CAD build for the part. Positions are in the model's coordinates, mm. Coordinates: 2 decimals unless noted, no trailing zeros. Loops run counter-clockwise (first coordinate to the right, second up) from the corner with the lowest first, then second, coordinate; pieces in that order, holes last. Notation, with made-up numbers: (16.25, -33.75) -> (49.25, -33.75) arc R16 ccw to (49.25, -26.75) -> close; hole circle Ø4 at (51.25, 31). An arc over 180 degrees is marked (long way). Answer as a JSON object with one key per item and string values. Group by question number.
from build123d import *

# Parameters (mm, degrees)
SKETCH1_W           = 256
SKETCH1_H           = 360
BOSS_EXTRUDE1_DEPTH = 3
FILLET1_R           = 2
SKETCH2_R           = 4
CUT_EXTRUDE2_DEPTH  = 221.89137602
SKETCH4_R           = 2.05
CUT_EXTRUDE3_DEPTH  = 221.89137602
SKETCH5_R           = 2.05
CUT_EXTRUDE4_DEPTH  = 221.89137602
CUT_EXTRUDE5_DEPTH  = 221.89137602


with BuildPart() as part:
    # Sketch1 → Boss-Extrude1 (new body)
    with BuildSketch(Plane(origin=(0, 0, 0), x_dir=(1, 0, 0), z_dir=(0, 1, 0))):
        Rectangle(SKETCH1_W, SKETCH1_H)
    extrude(amount=-BOSS_EXTRUDE1_DEPTH)

    # Fillet1
    fillet1_edges = [part.edges().sort_by_distance(p)[0] for p in [
        (-128, -1.5, -180),
        (128, -1.5, -180),
        (128, -1.5, 180),
        (-128, -1.5, 180),
    ]]
    fillet(fillet1_edges, radius=FILLET1_R)

    # Sketch2 → Cut-Extrude2 (cut, through all)
    with BuildSketch(Plane(origin=(0, 0, 0), x_dir=(1, 0, 0), z_dir=(0, 1, 0))):
        with Locations(Location((-120, 104, 0), (0, 0, 270))):
            Circle(SKETCH2_R)
        with Locations(Location((-120, 120, 0), (0, 0, 270))):
            Circle(SKETCH2_R)
        with Locations(Location((120, 104, 0), (0, 0, 90))):
            Circle(SKETCH2_R)
        with Locations(Location((120, 120, 0), (0, 0, 90))):
            Circle(SKETCH2_R)
        with Locations(Location((120, -104, 0), (0, 0, 270))):
            Circle(SKETCH2_R)
        with Locations(Location((120, -120, 0), (0, 0, 270))):
            Circle(SKETCH2_R)
        with Locations(Location((-120, -120, 0), (0, 0, 90))):
            Circle(SKETCH2_R)
        with Locations(Location((-120, -104, 0), (0, 0, 90))):
            Circle(SKETCH2_R)
    extrude(amount=-CUT_EXTRUDE2_DEPTH, mode=Mode.SUBTRACT)

    # Sketch4 → Cut-Extrude3 (cut, through all)
    with BuildSketch(Plane(origin=(0, 0, 0), x_dir=(1, 0, 0), z_dir=(0, 1, 0))):
        with Locations(Location((-120, 168, 0), (0, 0, 270))):
            Circle(SKETCH4_R)
        with Locations(Location((-104, 168, 0), (0, 0, 270))):
            Circle(SKETCH4_R)
        with Locations(Location((-56, 168, 0), (0, 0, 270))):
            Circle(SKETCH4_R)
        with Locations(Location((-8, 168, 0), (0, 0, 270))):
            Circle(SKETCH4_R)
        with Locations(Location((-104, 152, 0), (0, 0, 270))):
            Circle(SKETCH4_R)
        with Locations(Location((-104, 120, 0), (0, 0, 270))):
            Circle(SKETCH4_R)
        with Locations(Location((-104, 104, 0), (0, 0, 270))):
            Circle(SKETCH4_R)
        with Locations(Location((-8, 88, 0), (0, 0, 270))):
            Circle(SKETCH4_R)
        with Locations(Location((-104, 56, 0), (0, 0, 270))):
            Circle(SKETCH4_R)
        with Locations(Location((-104, 8, 0), (0, 0, 270))):
            Circle(SKETCH4_R)
        with Locations(Location((-88, 8, 0), (0, 0, 270))):
            Circle(SKETCH4_R)
        with Locations(Location((-120, 152, 0), (0, 0, 270))):
            Circle(SKETCH4_R)
        with Locations((-120, 120)):
            Circle(SKETCH4_R)
        with Locations((-120, 104)):
            Circle(SKETCH4_R)
        with Locations(Location((-120, 56, 0), (0, 0, 270))):
            Circle(SKETCH4_R)
        with Locations(Location((-120, 8, 0), (0, 0, 270))):
            Circle(SKETCH4_R)
        with Locations(Location((120, 8, 0), (0, 0, 90))):
            Circle(SKETCH4_R)
        with Locations(Location((120, 56, 0), (0, 0, 90))):
            Circle(SKETCH4_R)
        with Locations((120, 104)):
            Circle(SKETCH4_R)
        with Locations((120, 120)):
            Circle(SKETCH4_R)
        with Locations(Location((120, 152, 0), (0, 0, 90))):
            Circle(SKETCH4_R)
        with Locations(Location((88, 8, 0), (0, 0, 90))):
            Circle(SKETCH4_R)
        with Locations(Location((104, 8, 0), (0, 0, 90))):
            Circle(SKETCH4_R)
        with Locations(Location((104, 56, 0), (0, 0, 90))):
            Circle(SKETCH4_R)
        with Locations(Location((8, 88, 0), (0, 0, 90))):
            Circle(SKETCH4_R)
        with Locations(Location((104, 104, 0), (0, 0, 90))):
            Circle(SKETCH4_R)
        with Locations(Location((104, 120, 0), (0, 0, 90))):
            Circle(SKETCH4_R)
        with Locations(Location((104, 152, 0), (0, 0, 90))):
            Circle(SKETCH4_R)
        with Locations(Location((8, 168, 0), (0, 0, 90))):
            Circle(SKETCH4_R)
        with Locations(Location((56, 168, 0), (0, 0, 90))):
            Circle(SKETCH4_R)
        with Locations(Location((104, 168, 0), (0, 0, 90))):
            Circle(SKETCH4_R)
        with Locations(Location((120, 168, 0), (0, 0, 90))):
            Circle(SKETCH4_R)
        with Locations(Location((120, -168, 0), (0, 0, 270))):
            Circle(SKETCH4_R)
        with Locations(Location((104, -168, 0), (0, 0, 270))):
            Circle(SKETCH4_R)
        with Locations(Location((56, -168, 0), (0, 0, 270))):
            Circle(SKETCH4_R)
        with Locations(Location((8, -168, 0), (0, 0, 270))):
            Circle(SKETCH4_R)
        with Locations(Location((104, -152, 0), (0, 0, 270))):
            Circle(SKETCH4_R)
        with Locations(Location((104, -120, 0), (0, 0, 270))):
            Circle(SKETCH4_R)
        with Locations(Location((104, -104, 0), (0, 0, 270))):
            Circle(SKETCH4_R)
        with Locations(Location((8, -88, 0), (0, 0, 270))):
            Circle(SKETCH4_R)
        with Locations(Location((104, -56, 0), (0, 0, 270))):
            Circle(SKETCH4_R)
        with Locations(Location((104, -8, 0), (0, 0, 270))):
            Circle(SKETCH4_R)
        with Locations(Location((88, -8, 0), (0, 0, 270))):
            Circle(SKETCH4_R)
        with Locations(Location((120, -152, 0), (0, 0, 270))):
            Circle(SKETCH4_R)
        with Locations((120, -120)):
            Circle(SKETCH4_R)
        with Locations((120, -104)):
            Circle(SKETCH4_R)
        with Locations(Location((120, -56, 0), (0, 0, 270))):
            Circle(SKETCH4_R)
        with Locations(Location((120, -8, 0), (0, 0, 270))):
            Circle(SKETCH4_R)
        with Locations(Location((-120, -8, 0), (0, 0, 90))):
            Circle(SKETCH4_R)
        with Locations(Location((-120, -56, 0), (0, 0, 90))):
            Circle(SKETCH4_R)
        with Locations((-120, -104)):
            Circle(SKETCH4_R)
        with Locations((-120, -120)):
            Circle(SKETCH4_R)
        with Locations(Location((-120, -152, 0), (0, 0, 90))):
            Circle(SKETCH4_R)
        with Locations(Location((-88, -8, 0), (0, 0, 90))):
            Circle(SKETCH4_R)
        with Locations(Location((-104, -8, 0), (0, 0, 90))):
            Circle(SKETCH4_R)
        with Locations(Location((-104, -56, 0), (0, 0, 90))):
            Circle(SKETCH4_R)
        with Locations(Location((-8, -88, 0), (0, 0, 90))):
            Circle(SKETCH4_R)
        with Locations(Location((-104, -104, 0), (0, 0, 90))):
            Circle(SKETCH4_R)
        with Locations(Location((-104, -120, 0), (0, 0, 90))):
            Circle(SKETCH4_R)
        with Locations(Location((-104, -152, 0), (0, 0, 90))):
            Circle(SKETCH4_R)
        with Locations(Location((-8, -168, 0), (0, 0, 90))):
            Circle(SKETCH4_R)
        with Locations(Location((-56, -168, 0), (0, 0, 90))):
            Circle(SKETCH4_R)
        with Locations(Location((-104, -168, 0), (0, 0, 90))):
            Circle(SKETCH4_R)
        with Locations(Location((-120, -168, 0), (0, 0, 90))):
            Circle(SKETCH4_R)
    extrude(amount=-CUT_EXTRUDE3_DEPTH, mode=Mode.SUBTRACT)

    # Sketch5 → Cut-Extrude4 (cut, through all)
    with BuildSketch(Plane(origin=(0, 0, 0), x_dir=(1, 0, 0), z_dir=(0, 1, 0))):
        with Locations(Location((-112, 90.15, 0), (0, 0, 270))):
            Circle(SKETCH5_R)
        with Locations(Location((-90, 112, 0), (0, 0, 270))):
            Circle(SKETCH5_R)
        with Locations(Location((112, 90.15, 0), (0, 0, 90))):
            Circle(SKETCH5_R)
        with Locations(Location((90, 112, 0), (0, 0, 90))):
            Circle(SKETCH5_R)
        with Locations(Location((112, -90.15, 0), (0, 0, 270))):
            Circle(SKETCH5_R)
        with Locations(Location((90, -112, 0), (0, 0, 270))):
            Circle(SKETCH5_R)
        with Locations(Location((-90, -112, 0), (0, 0, 90))):
            Circle(SKETCH5_R)
        with Locations(Location((-112, -90.15, 0), (0, 0, 90))):
            Circle(SKETCH5_R)
    extrude(amount=-CUT_EXTRUDE4_DEPTH, mode=Mode.SUBTRACT)

    # Sketch6 → Cut-Extrude5 (cut, through all)
    with BuildSketch(Plane(origin=(0, 0, 0), x_dir=(1, 0, 0), z_dir=(0, 1, 0))):
        with BuildLine():
            Line((-72, 122), (72, 122))
            ThreePointArc((72, 122), (74, 120), (72, 118))
            Line((72, 118), (-72, 118))
            ThreePointArc((-72, 118), (-74, 120), (-72, 122))
        make_face()
        with BuildLine():
            Line((-72, 106), (72, 106))
            ThreePointArc((72, 106), (74, 104), (72, 102))
            Line((72, 102), (-72, 102))
            ThreePointArc((-72, 102), (-74, 104), (-72, 106))
        make_face()
        with BuildLine():
            Line((-10, -56), (-10, 56))
            ThreePointArc((-10, 56), (-8, 58), (-6, 56))
            Line((-6, 56), (-6, -56))
            ThreePointArc((-6, -56), (-8, -58), (-10, -56))
        make_face()
        with BuildLine():
            Line((-42, -56), (-42, 56))
            ThreePointArc((-42, 56), (-40, 58), (-38, 56))
            Line((-38, 56), (-38, -56))
            ThreePointArc((-38, -56), (-40, -58), (-42, -56))
        make_face()
        with BuildLine():
            Line((-74, -56), (-74, 56))
            ThreePointArc((-74, 56), (-72, 58), (-70, 56))
            Line((-70, 56), (-70, -56))
            ThreePointArc((-70, -56), (-72, -58), (-74, -56))
        make_face()
        with BuildLine():
            Line((-72, -106), (72, -106))
            ThreePointArc((72, -106), (74, -104), (72, -102))
            Line((72, -102), (-72, -102))
            ThreePointArc((-72, -102), (-74, -104), (-72, -106))
        make_face()
        with BuildLine():
            Line((-72, -122), (72, -122))
            ThreePointArc((72, -122), (74, -120), (72, -118))
            Line((72, -118), (-72, -118))
            ThreePointArc((-72, -118), (-74, -120), (-72, -122))
        make_face()
        with BuildLine():
            Line((74, -56), (74, 56))
            ThreePointArc((74, 56), (72, 58), (70, 56))
            Line((70, 56), (70, -56))
            ThreePointArc((70, -56), (72, -58), (74, -56))
        make_face()
        with BuildLine():
            Line((42, -56), (42, 56))
            ThreePointArc((42, 56), (40, 58), (38, 56))
            Line((38, 56), (38, -56))
            ThreePointArc((38, -56), (40, -58), (42, -56))
        make_face()
        with BuildLine():
            Line((10, -56), (10, 56))
            ThreePointArc((10, 56), (8, 58), (6, 56))
            Line((6, 56), (6, -56))
            ThreePointArc((6, -56), (8, -58), (10, -56))
        make_face()
    extrude(amount=-CUT_EXTRUDE5_DEPTH, mode=Mode.SUBTRACT)


solid = part.part
Item 1: Band-saw the part on B-B, the plane y = -1. Count the separate pieces of the cut face and the enclosed holes in it, and give its area (3 significant figures).
Item 2: Band-saw the part on A-A, the plane z = -40. List the corners of the cut face in (x, y).
Item 3: Drill centre lines: L1, parallel to X at y = -0.8, z = -104; L2, parallel to Z at x = -68.5, y = -2.2; L3, parallel to X at y = -0.9, z = -101.5. Where is each one in solid material? Low to high.
Item 4: Pull direction Z, two halves, no side cores. Call faces 1 (the cylindrical face through (-116.034, -1.479, -104.521)), 2 (the flat face through (-2, 0, -3)), 3 (the cylindrical face through (116.034, -1.479, -103.479)): +Z half, -Z half, draft (parallel to the pull), parting line (faces both ways), or undercut.
Reply:
{
 "1": {"separate pieces": "1", "enclosed holes": "82", "area": "85,800 mm²"},
 "2": {"outline": "(-128, -3) -> (-74, -3) -> (-74, 0) -> (-128, 0) -> close; (-70, -3) -> (-42, -3) -> (-42, 0) -> (-70, 0) -> close; (-38, -3) -> (-10, -3) -> (-10, 0) -> (-38, 0) -> close; (-6, -3) -> (6, -3) -> (6, 0) -> (-6, 0) -> close; (10, -3) -> (38, -3) -> (38, 0) -> (10, 0) -> close; (42, -3) -> (70, -3) -> (70, 0) -> (42, 0) -> close; (74, -3) -> (128, -3) -> (128, 0) -> (74, 0) -> close"},
 "3": {"L1": "-128 to -124, -116 to -106.05, -101.95 to -74, 74 to 101.95, 106.05 to 116, 124 to 128", "L2": "-180 to -122, -118 to -106, -102 to 102, 106 to 118, 122 to 180", "L3": "-128 to -123.12, -116.88 to 116.88, 123.12 to 128"},
 "4": {"face 1": "undercut", "face 2": "draft", "face 3": "undercut"}
}
